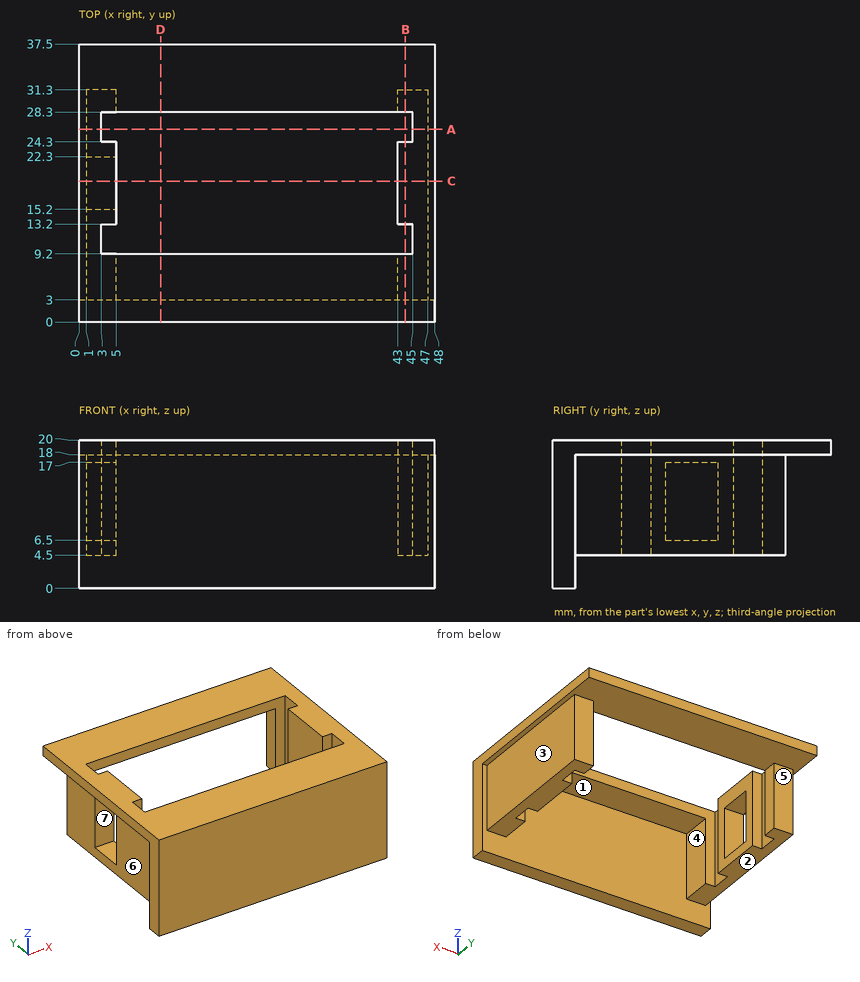
Source: three-view drawing plus pictorial views. Frame: mm from the lowest corner of the part. A direction names the side the tool comes from. Coordinates: 2 decimals unless noted, no trailing zeros. Write each loop counter-clockwise with the first axis right and the second up, starting at its lowest first coordinate (ties: lowest second). Pieces come first, ordered by that corner, then holes. Notation, with made-up numbers: (-9, 0) - (40, 0) arc R27 cw to (40, 26) - close; hole circle Ø2 at (80.5, 68). An arc over 180 degrees is marked (long way). Answer as a JSON object with one key per item and string values.
Q1. Section query B-B, the plane x = 44. Output: boundary loops of the cut face in (y, z).
Ans:
{"outline": "(0, 0) - (3, 0) - (3, 4.5) - (9.2, 4.5) - (9.2, 20) - (0, 20) - close; (13.2, 4.5) - (24.3, 4.5) - (24.3, 20) - (13.2, 20) - close; (28.3, 4.5) - (31.3, 4.5) - (31.3, 18) - (37.5, 18) - (37.5, 20) - (28.3, 20) - close"}
Q2. Draft query along X for the marked faces 1, 2 and 3. Return one class per face: released by +X, released by -X, zero draft, split by the parting line, or undercut.
Ans:
{"face 1": "undercut", "face 2": "zero draft", "face 3": "released by +X"}
Q3. Section query C-C, the plane y = 19. Output: boundary loops of the cut face in (x, z).
Ans:
{"outline": "(0, 18) - (1, 18) - (1, 17) - (5, 17) - (5, 20) - (0, 20) - close; (1, 4.5) - (5, 4.5) - (5, 6.5) - (1, 6.5) - close; (43, 4.5) - (47, 4.5) - (47, 18) - (48, 18) - (48, 20) - (43, 20) - close"}
Q4. Material intervals for line 1 (Y direction, x = 4.5, z = 16.5); line 2 (Y direction, x = 44.5, z = 15.5); line 3 (Y direction, x = 33.5, z = 18.25), sorted ascending. Write a range as [from, to].
Ans:
{"line 1": "y = [0, 9.2], [13.2, 15.2], [22.3, 24.3], [28.3, 31.3]", "line 2": "y = [0, 9.2], [13.2, 24.3], [28.3, 31.3]", "line 3": "y = [0, 9.2], [28.3, 37.5]"}
Q5. Section query D-D, the plane x = 11. Output: boundary loops of the cut face in (y, z).
Ans:
{"outline": "(0, 0) - (3, 0) - (3, 18) - (9.2, 18) - (9.2, 20) - (0, 20) - close; (28.3, 18) - (37.5, 18) - (37.5, 20) - (28.3, 20) - close"}
Q6. Set-up query: the marked faces 4, 5, 6 and 7. Return all of +Z, -Z, +X, -X, +Y, -Y with unobstructed straight access to the full face (end or side cutting, diameter ignored); none if empty.
Ans:
{"face 4": "-Z, +Y", "face 5": "-Z, +X, -X, +Y", "face 6": "-Z, -X, +Y", "face 7": "-X"}
Q7. First-contact query: pin 1 Ø3 at (y, z) = (5.5, 11) entering from -X; pin 2 Ø1.2 at (x, y) = (4, 17.5) entering from -Z; pin 3 Ø1.9 at (x, y) = (29, 7) entering from -Z. Flat tips, straight axial feed; report the tip coordinate or a pass-through.
Ans:
{"pin 1": "stops at x = 1", "pin 2": "stops at z = 4.5", "pin 3": "stops at z = 18"}
Q8. Section query A-A, the plane y = 26. Output: boundary loops of the cut face in (x, z).
Ans:
{"outline": "(0, 18) - (1, 18) - (1, 4.5) - (3, 4.5) - (3, 20) - (0, 20) - close; (45, 4.5) - (47, 4.5) - (47, 18) - (48, 18) - (48, 20) - (45, 20) - close"}
